Can you work these out from the model? Positions are in its coordinate system, mm. Coordinates: 2 decimals unless noted, no trailing zeros. Order: outer loops, then holes, each group sorted by start corner. A loop starts at its lowest first (then second) coordinate and runs counter-clockwise, first axis right, second up. Notation, with made-up numbers: (53.5, -8) - (62.5, -8) arc R15 cw to (62.5, 18) - close; hole circle Ø5 at (74, 40.5). An arc over 180 degrees is marked (long way). Return JSON: item names as keys, results as strings. Group by question number.
1) Imagine slicing it at D-D (x = -24.5). Write out the boundary of the cut face in (y, z).
2) If I drill on line 1 along Y through (x, z) = (1.5, 1.8); line 2 along Y through (x, z) = (-24, 1.9); line 3 along X through (y, z) = (-17.5, 4.5), over which ranges is the centre line in solid material (lowest first)?
3) Imagine slicing it at C-C (y = 27.5). Write out the boundary of the cut face in (x, z).
4) For pin 1 Ø3 at (x, y) = (0, -27.5) entering from -Z; pin 2 Ø2 at (y, z) = (7, 1) entering from -X; pin 3 Ø2 at (y, z) = (-19.5, 3.5) entering from +X; pin 4 Ø3 at (x, z) = (6.5, 4) entering from +Y, each with a flat end and sliding along its axis, tell me the tip position at first contact or that it passes through.
5) Imagine slicing it at A-A (y = 0). Write out the boundary of the cut face in (x, z), and give its area (3 significant figures).
```python
from build123d import *

# Parameters (mm, degrees)
SKETCH1_R           = 30
SKETCH1_R_2         = 1.75
SKETCH1_R_3         = 2.5
BOSS_EXTRUDE1_DEPTH = 5


with BuildPart() as part:
    # Sketch1 → Boss-Extrude1 (new body)
    with BuildSketch(Plane.XY):
        Circle(SKETCH1_R)
        with Locations((0, 27.5)):
            Circle(SKETCH1_R_2, mode=Mode.SUBTRACT)
        with Locations((27.5, 0)):
            Circle(SKETCH1_R_2, mode=Mode.SUBTRACT)
        with Locations((0, -27.5)):
            Circle(SKETCH1_R_2, mode=Mode.SUBTRACT)
        with Locations((-27.5, 0)):
            Circle(SKETCH1_R_2, mode=Mode.SUBTRACT)
        with Locations((6.278593331, 24.198745128)):
            Circle(SKETCH1_R_3, mode=Mode.SUBTRACT)
        with Locations((17.817431356, -17.536793889)):
            Circle(SKETCH1_R_3, mode=Mode.SUBTRACT)
        with Locations((-24.096024686, -6.66195124)):
            Circle(SKETCH1_R_3, mode=Mode.SUBTRACT)
    extrude(amount=BOSS_EXTRUDE1_DEPTH)


solid = part.part
```
Calculated:
{
 "1": {"outline": "(-17.31, 0) - (-9.13, 0) - (-9.13, 5) - (-17.31, 5) - close; (-4.19, 0) - (17.31, 0) - (17.31, 5) - (-4.19, 5) - close"},
 "2": {"line 1": "-29.96 to -28.4, -26.6 to 26.6, 28.4 to 29.96", "line 2": "-18 to -9.16, -4.16 to 18", "line 3": "-24.37 to 15.32, 20.32 to 24.37"},
 "3": {"outline": "(-11.99, 0) - (-1.75, 0) - (-1.75, 5) - (-11.99, 5) - close; (1.75, 0) - (11.99, 0) - (11.99, 5) - (1.75, 5) - close"},
 "4": {"pin 1": "through", "pin 2": "x = -29.39", "pin 3": "x = 23.62", "pin 4": "y = 29.58"},
 "5": {"outline": "(-30, 0) - (-29.25, 0) - (-29.25, 5) - (-30, 5) - close; (-25.75, 0) - (25.75, 0) - (25.75, 5) - (-25.75, 5) - close; (29.25, 0) - (30, 0) - (30, 5) - (29.25, 5) - close", "area": "265 mm2"}
}
